Part model, mm, in its own coordinate system. A direction names the side the tool comes from. Coordinates: 2 decimals unless noted, no trailing zeros. Order: outer loops, then holes, each group sorted by start corner. A loop starts at its lowest first (then second) coordinate and runs counter-clockwise, first axis right, second up.
```python
from build123d import *

# Parameters (mm, degrees)
PAD002_DEPTH      = 5
PAD002_DEPTH_BACK = 100
SKETCH002_R       = 2
SKETCH002_R_2     = 2.000137
PAD001_DEPTH      = 17.5
SKETCH_R          = 12.5459
SKETCH_R_2        = 8
PAD_DEPTH         = 20
PAD_DEPTH_BACK    = 50


with BuildPart() as pad002:
    # Sketch003 → Pad002 (new body, two sides)
    with BuildSketch(Plane.XY) as pad002_sk:
        Polygon((1, 0), (13, 12), (12, 13), (0, 1), (-12, 13), (-13, 12), (-1, 0), (-12, -11), (-11, -12), (0, -1), (11, -12), (12, -11), align=None)
    extrude(amount=PAD002_DEPTH)
    extrude(pad002_sk.sketch, amount=-PAD002_DEPTH_BACK)


with BuildPart() as pad001:
    # Sketch002 → Pad001 (new body, symmetric)
    with BuildSketch(Plane.XZ):
        with Locations((0, 14)):
            Circle(SKETCH002_R)
        with Locations((0, -44.638561)):
            Circle(SKETCH002_R_2)
    extrude(amount=PAD001_DEPTH, both=True)


with BuildPart() as revolution:
    # Sketch001 → Revolution (revolve)
    with BuildSketch(Plane.XZ):
        with BuildLine():
            Line((-10, 0), (-25.954499, 0))
            Line((-25.954499, 0), (-25.954499, -3.694792))
            Line((-25.954499, -3.694792), (-15.790939, -3.694792))
            ThreePointArc((-12.482958, -7.002773), (-13.451843, -4.663677), (-15.790939, -3.694792))
            Line((-12.482958, -7.002773), (-12.482958, -17.250204))
            Line((-12.482958, -17.250204), (-10, -17.250204))
            Line((-10, -17.250204), (-10, 0))
        make_face()
    revolve(axis=Axis((0, 0, 0), (0, 0, 1)))


with BuildPart() as cut001:
    # Sketch → Pad (new body, two sides)
    with BuildSketch(Plane.XY) as pad_sk:
        Circle(SKETCH_R)
        Circle(SKETCH_R_2, mode=Mode.SUBTRACT)
    extrude(amount=PAD_DEPTH)
    extrude(pad_sk.sketch, amount=-PAD_DEPTH_BACK)

    # Fusion: union Revolution
    add(revolution.part)

    # Cut: cut Pad001
    add(pad001.part, mode=Mode.SUBTRACT)

    # Cut001: cut Pad002
    add(pad002.part, mode=Mode.SUBTRACT)


solid = cut001.part
```
(1) Probe line 1 (Z direction, x = 0, y = 9.7); line 2 (X direction, y = 0, z = -6.5); line 3 (Y direction, x = 0, z = -1). List the from-to ranges inside material, lowest first.
(2) Drop flat-ended pins along their axis: pin 1 (1.5 mm diameter, centred on x = 5.5, z = -23, fed in from -Y); pin 2 (6 mm diameter, centred on x = 17, z = 1.5, fed in from +Y); pin 3 (1.5 mm diameter, centred on y = 15, z = -13.5, fed in from -X) (3 decimals); pin 4 (4.5 mm diameter, centred on x = 0, z = 14, fed in from -Y). Give the stop position or say it passes through.
(3) Slice it at B-B, the plane x = 0. State how many separate pieces and enclosed holes the cut face has, then the cut area to 3 significant figures.
(4) Tool access for faces 4 (the face through (-8, -7, -22)), 5 (the face through (-12.545, 0.128, -27.875)), 6 (the face through (-0.128, -12.545, -27.875)), 7 (the face through (12.545, -0.128, -27.875)), 8 (the face through (5.79, -11.13, 10.14)): list every direction of +Z, -Z, +X, -X, +Y, -Y with a clear straight run to the whole face (end or side of a thin tool).
(5) Pull direction Y, two halves, no side cores. Call faces 1 (the face through (8, 7, -22)), 2 (the face through (1.908, -10.111, 14.601)), 3 (the face through (3.379, -25.734, -1.873)): +Y half, -Y half, draft (parallel to the pull), parting line (faces both ways), or undercut.
(6) Slice it at C-C, the plane z = -1.5. Give the cut face in (x, y).
(7) Slice it at A-A, the plane y = 0. Give the cut face in (x, z), then the cut area to 3 significant figures.
(8) Slice it at D-D, the plane z = -33.5. Give the cut face in (x, y), then the cut area to 3 significant figures.
Here are the results:
1. line 1: z = -50 to -46.64, -42.64 to 12, 16 to 20
1. line 2: x = -12.55 to -8, 8 to 12.55
1. line 3: y = -25.95 to -8, 8 to 25.95
2. pin 1: stops at y = -11.61
2. pin 2: stops at y = 21.59
2. pin 3: passes through
2. pin 4: stops at y = -12.55
3. separate pieces: 6
3. enclosed holes: 0
3. area: 667 mm2
4. face 4: -Z
4. face 5: -Z, -X
4. face 6: -Z, -Y
4. face 7: -Z, +X
4. face 8: +Z
5. face 1: undercut
5. face 2: draft
5. face 3: parting line
6. outline: circle Ø51.91 at (0, 0); hole (-13, 12) - (-6.13, 5.13) arc R8 ccw to (-6.13, -5.13) - (-12, -11) - (-11, -12) - (-5.13, -6.13) arc R8 ccw to (5.13, -6.13) - (11, -12) - (12, -11) - (6.13, -5.13) arc R8 ccw to (6.13, 5.13) - (13, 12) - (12, 13) - (5.13, 6.13) arc R8 ccw to (-5.13, 6.13) - (-12, 13) - close
7. outline: (-25.95, -3.69) - (-15.79, -3.69) arc R3.31 cw to (-12.55, -6.36) - (-12.55, -50) - (-8, -50) - (-8, 20) - (-12.55, 20) - (-12.55, 0) - (-25.95, 0) - close; (8, -50) - (12.55, -50) - (12.55, -6.36) arc R3.31 cw to (15.79, -3.69) - (25.95, -3.69) - (25.95, 0) - (12.55, 0) - (12.55, 20) - (8, 20) - close
7. area: 740 mm2
8. outline: (-9.36, -8.36) - (-6.13, -5.13) arc R8 cw to (-6.13, 5.13) - (-9.36, 8.36) arc R12.55 ccw to start; (-8.36, -9.36) arc R12.55 ccw to (8.36, -9.36) - (5.13, -6.13) arc R8 cw to (-5.13, -6.13) - close; (-8.36, 9.36) - (-5.13, 6.13) arc R8 cw to (5.13, 6.13) - (8.36, 9.36) arc R12.55 ccw to start; (6.13, -5.13) - (9.36, -8.36) arc R12.55 ccw to (9.36, 8.36) - (6.13, 5.13) arc R8 cw to start
8. area: 268 mm2
